```python
from build123d import *

# Parameters (mm, degrees)
SKETCH1_W                                         = 20.32
SKETCH1_H                                         = 76.2
BOSS_EXTRUDE1_DEPTH                               = 5.08
CSK_FOR_6_FLAT_HEAD_MACHINE_SCREW_100_D           = 4.3053
CSK_FOR_6_FLAT_HEAD_MACHINE_SCREW_100_CSINK_D     = 8.297418
CSK_FOR_6_FLAT_HEAD_MACHINE_SCREW_100_CSINK_ANGLE = 100
FILLET1_R                                         = 2.54


with BuildPart() as part:
    # Sketch1 → Boss-Extrude1 (new body)
    with BuildSketch(Plane(origin=(0, 0, 0), x_dir=(1, 0, 0), z_dir=(0, 1, 0))):
        Rectangle(SKETCH1_W, SKETCH1_H)
    extrude(amount=BOSS_EXTRUDE1_DEPTH)

    # CSK for #6 Flat Head Machine Screw (100)1 (through all)
    with Locations(Plane(origin=(0, 5.08, 0), x_dir=(1, 0, 0), z_dir=(0, 1, 0))):
        with Locations((0, 31.75)):
            CounterSinkHole(CSK_FOR_6_FLAT_HEAD_MACHINE_SCREW_100_D / 2, CSK_FOR_6_FLAT_HEAD_MACHINE_SCREW_100_CSINK_D / 2, counter_sink_angle=CSK_FOR_6_FLAT_HEAD_MACHINE_SCREW_100_CSINK_ANGLE)

    # Fillet1
    # the kernel refuses this fillet: 2.54 mm, written as the material it takes off along each edge
    with BuildSketch(Plane(origin=(-10.16, 5.08, -44.45), x_dir=(1, 0, 0), z_dir=(0, 0, 1)), Plane(origin=(10.16, 5.08, 44.45), x_dir=(-1, 0, 0), z_dir=(0, 0, -1))) as fillet1_piece_1:
        with BuildLine():
            CenterArc((FILLET1_R, -FILLET1_R), FILLET1_R, 90, 90)
            Line((0, -FILLET1_R), (0, 0))
            Line((0, 0), (FILLET1_R, 0))
        make_face()
    extrude(amount=88.9, mode=Mode.SUBTRACT)
    with BuildSketch(Plane(origin=(-16.51, 5.08, 38.1), x_dir=(0, -1, 0), z_dir=(1, 0, 0))) as fillet1_piece_2:
        with BuildLine():
            CenterArc((FILLET1_R, FILLET1_R), FILLET1_R, 180, 90)
            Line((0, FILLET1_R), (0, 0))
            Line((0, 0), (FILLET1_R, 0))
        make_face()
    extrude(amount=33.02, mode=Mode.SUBTRACT)
    with BuildSketch(Plane(origin=(16.51, 5.08, -38.1), x_dir=(0, 0, 1), z_dir=(-1, 0, 0))) as fillet1_piece_3:
        with BuildLine():
            CenterArc((FILLET1_R, -FILLET1_R), FILLET1_R, 90, 90)
            Line((0, -FILLET1_R), (0, 0))
            Line((0, 0), (FILLET1_R, 0))
        make_face()
    extrude(amount=33.02, mode=Mode.SUBTRACT)


solid = part.part
```
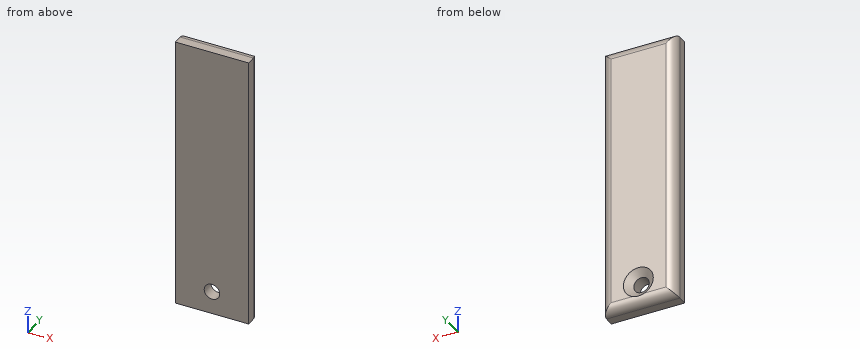
For this review, take the finished solid that the model builds, in its own axes (mm). Round coordinates to 2 decimals unless told otherwise and drop trailing zeros. Write each loop counter-clockwise with the first axis right and the second up, starting at its lowest first coordinate (ties: lowest second). Pieces come first, ordered by that corner, then holes. Notation, with made-up numbers: (-6.5, -17) - (27.5, -17) arc R15 ccw to (27.5, 2) - close; hole circle Ø8 at (65, 51.5). An arc over 180 degrees is marked (long way). Put each result on its own line as item: value.
Q1. We need section C-C (y = 4.35). Give the boundary of the cut face in (x, z), and give its area (3 significant figures).
Solved:
outline: (-9.4, -37.34) - (9.4, -37.34) - (9.4, 37.34) - (-9.4, 37.34) - close; hole circle Ø6.56 at (0, -31.75)
area: 1,370 mm2
Q2. We need section A-A (z = -31.75). Give the boundary of the cut face in (x, y).
Solved:
outline: (-10.16, 0) - (-2.15, 0) - (-2.15, 3.41) - (-4.15, 5.08) - (-7.62, 5.08) arc R2.54 ccw to (-10.16, 2.54) - close; (2.15, 0) - (10.16, 0) - (10.16, 2.54) arc R2.54 ccw to (7.62, 5.08) - (4.15, 5.08) - (2.15, 3.41) - close
Q3. We need section B-B (x = 0). Give the boundary of the cut face in (y, z).
Solved:
outline: (0, -38.1) - (2.54, -38.1) arc R2.54 ccw to (5.06, -35.88) - (3.41, -33.9) - (0, -33.9) - close; (0, -29.6) - (3.41, -29.6) - (5.08, -27.6) - (5.08, 35.56) arc R2.54 ccw to (2.54, 38.1) - (0, 38.1) - close
Q4. Wall thickness on probe 1 along Z at (x, y) = (0, 1.6); probe 2 along X at (y, z) = (2.45, -31.75); probe 3 along Z at (x, y) = (-0.5, 3.85): over which ranges is each line inside the solid? List them lowest first.
Solved:
probe 1: z = -38.1 to -33.9, -29.6 to 38.1
probe 2: x = -10.16 to -2.15, 2.15 to 10.16
probe 3: z = -37.74 to -34.39, -29.11 to 37.74
Q5. Insertion check: pin 1 Ø1.5 at (x, y) = (-5, 4) entering from -Z; pin 2 Ø5 at (x, z) = (0, -31.75) entering from +Y. Each pin has a flat end and moves straight along its axis. Give the tip position at first contact, or say it passes through.
Solved:
pin 1: stops at z = -38
pin 2: stops at y = 3.7
Q6. We need section D-D (z = 20.5). Give the boundary of the cut face in (x, y).
Solved:
outline: (-10.16, 0) - (10.16, 0) - (10.16, 2.54) arc R2.54 ccw to (7.62, 5.08) - (-7.62, 5.08) arc R2.54 ccw to (-10.16, 2.54) - close
